from build123d import *

# Parameters (mm, degrees)
SKETCH_W        = 32
SKETCH_H        = 40
PAD_DEPTH       = 6
CHAMFER_SIZE    = 4
CHAMFER001_SIZE = 1
SKETCH001_W     = 20.25
SKETCH001_H     = 20
POCKET_DEPTH    = 10


with BuildPart() as part:
    # Sketch (on XY_Plane of Origin) → Pad (new body)
    with BuildSketch(Plane.XY):
        Rectangle(SKETCH_W, SKETCH_H)
    extrude(amount=PAD_DEPTH)

    # Chamfer
    chamfer_edges = [part.edges().sort_by_distance(p)[0] for p in [
        (16, 20, 3),
        (16, -20, 3),
        (-16, 20, 3),
        (-16, -20, 3),
    ]]
    chamfer(chamfer_edges, length=CHAMFER_SIZE)

    # Chamfer001
    chamfer001_edges = [part.edges().sort_by_distance(p)[0] for p in [
        (0, -20, 0),
        (0, -20, 6),
        (0, 20, 0),
        (0, 20, 6),
    ]]
    chamfer(chamfer001_edges, length=CHAMFER001_SIZE)

    # Sketch001 (on Face8 of Chamfer001) → Pocket (cut)
    with BuildSketch(Plane.XY.offset(6)):
        with Locations((0, -27.031727)):
            Rectangle(SKETCH001_W, SKETCH001_H)
        with Locations((0, 27.031727)):
            Rectangle(SKETCH001_W, SKETCH001_H)
    extrude(amount=-POCKET_DEPTH, mode=Mode.SUBTRACT)


solid = part.part
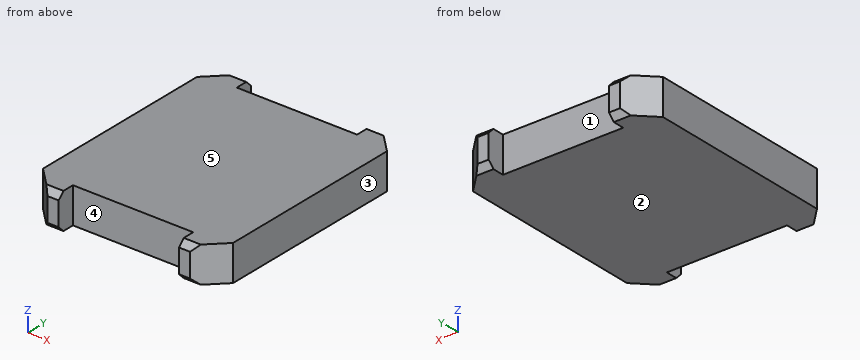
For this review, take the finished solid that the model builds, in its own axes (mm). Face numbers are marked on the shaded views. A direction names the side the tool comes from. Round coordinates to 2 decimals unless told otherwise and drop trailing zeros. Write each loop counter-clockwise with the first axis right and the second up, starting at its lowest first coordinate (ties: lowest second). Pieces come first, ordered by that corner, then holes. Notation, with made-up numbers: (46, 33) - (89, 33) arc R21 ccw to (89, 64) - close; hole circle Ø7 at (79.5, 86). An arc over 180 degrees is marked (long way). Use a Markdown table: item, result.
Q1. Wall thickness on line 1 along Y through (x, z) = (-4.5, 1); line 2 along X through (y, z) = (18.5, 3.75) (3 decimals); line 3 along Y through (x, z) = (-12.5, 2.75): over which ranges is each line inside the solid? List them lowest first.
Derived:
| item | result |
|---|---|
| line 1 | y = -17.03 to 17.03 |
| line 2 | x = -13.5 to -10.125, 10.125 to 13.5 |
| line 3 | y = -19.5 to 19.5 |
Q2. We need section B-B (x = 12.5). Give the boundary of the cut face in (y, z).
Derived:
| item | result |
|---|---|
| outline | (-19.5, 0.5) - (-19, 0) - (19, 0) - (19.5, 0.5) - (19.5, 5.5) - (19, 6) - (-19, 6) - (-19.5, 5.5) - close |
Q3. Clearance check with flat-ended pins moving along their axes: pin 1 (2.5 mm diameter, centred on y = 19, z = 2.5, fed in from +X); pin 2 (1.5 mm diameter, centred on y = 18, z = 2.5, fed in from -X); pin 3 (3.5 mm diameter, centred on y = -19, z = 4, fed in from +X). State where each tip first meets the part, or that it passes through.
Derived:
| item | result |
|---|---|
| pin 1 | stops at x = 14.25 |
| pin 2 | stops at x = -14.75 |
| pin 3 | stops at x = 14.75 |
Q4. We need section C-C (x = -6). Give the boundary of the cut face in (y, z), plus the area to 3 significant figures.
Derived:
| item | result |
|---|---|
| outline | (-17.03, 0) - (17.03, 0) - (17.03, 6) - (-17.03, 6) - close |
| area | 204 mm2 |
Q5. The part is to be moulded in two halves that separate along X. For the marked faces 1, 2 and 3, say which applies: pulls with the +X half, pulls with the -X half, needs draft (parallel to the pull), parting line crosses it, or undercut.
Derived:
| item | result |
|---|---|
| face 1 | undercut |
| face 2 | needs draft |
| face 3 | pulls with the +X half |
Q6. We need section A-A (z = 3). Give the boundary of the cut face in (x, y) (3 decimals).
Derived:
| item | result |
|---|---|
| outline | (-16, -16) - (-12, -20) - (-10.125, -20) - (-10.125, -17.032) - (10.125, -17.032) - (10.125, -20) - (12, -20) - (16, -16) - (16, 16) - (12, 20) - (10.125, 20) - (10.125, 17.032) - (-10.125, 17.032) - (-10.125, 20) - (-12, 20) - (-16, 16) - close |
Q7. Machinability: for the marked faces 4 and 5, which of the approach directions +Z, -Z, +X, -X, +Y, -Y give a long, thin tool a straight path to every point of the face, cutting with its end or side? Answer none if there is none.
Derived:
| item | result |
|---|---|
| face 4 | +Z, -Z, -Y |
| face 5 | +Z, +X, -X, +Y, -Y |
